```python
from build123d import *

# Parameters (mm, degrees)
SKETCH1_R           = 2.5
SKETCH1_R_2         = 1.75
SKETCH1_W           = 30
SKETCH1_H           = 6.4
BOSS_EXTRUDE1_DEPTH = 3.2


with BuildPart() as part:
    # Sketch1 → Boss-Extrude1 (new body)
    with BuildSketch(Plane(origin=(0, 0, 0), x_dir=(1, 0, 0), z_dir=(0, 1, 0))):
        Polygon((-87.5, 7.5), (-87.5, 20), (-84.3, 20), (-84.3, 35), (-87.5, 35), (-87.5, 50), (-70, 50), (-70, 46.8), (-50, 46.8), (-50, 50), (-30, 50), (-30, 46.8), (-10, 46.8), (-10, 50), (10, 50), (10, 46.8), (30, 46.8), (30, 50), (50, 50), (50, 46.8), (70, 46.8), (70, 50), (87.5, 50), (87.5, 35), (84.3, 35), (84.3, 20), (87.5, 20), (87.5, 7.5), (84.3, 7.5), (84.3, -7.5), (87.5, -7.5), (87.5, -20), (84.3, -20), (84.3, -35), (87.5, -35), (87.5, -50), (70, -50), (70, -46.8), (50, -46.8), (50, -50), (30, -50), (30, -46.8), (10, -46.8), (10, -50), (-10, -50), (-10, -46.8), (-30, -46.8), (-30, -50), (-50, -50), (-50, -46.8), (-70, -46.8), (-70, -50), (-87.5, -50), (-87.5, -35), (-84.3, -35), (-84.3, -20), (-87.5, -20), (-87.5, -7.5), (-84.3, -7.5), (-84.3, 7.5), align=None)
        with Locations((52.5, 15)):
            Circle(SKETCH1_R, mode=Mode.SUBTRACT)
        with Locations((42.34, 28)):
            Circle(SKETCH1_R_2, mode=Mode.SUBTRACT)
        with Locations((62.66, 28)):
            Circle(SKETCH1_R_2, mode=Mode.SUBTRACT)
        with Locations((62.66, -28)):
            Circle(SKETCH1_R_2, mode=Mode.SUBTRACT)
        with Locations((42.34, -28)):
            Circle(SKETCH1_R_2, mode=Mode.SUBTRACT)
        with Locations((52.5, -15)):
            Circle(SKETCH1_R, mode=Mode.SUBTRACT)
        with Locations((-54.3, 0)):
            Rectangle(SKETCH1_W, SKETCH1_H, mode=Mode.SUBTRACT)
    extrude(amount=BOSS_EXTRUDE1_DEPTH)


solid = part.part
```
Work out the finished part from the listing and answer in its coordinate system (mm). A direction names the side the tool comes from. Coordinates: 2 decimals unless noted, no trailing zeros. Loops run counter-clockwise (first coordinate to the right, second up) from the corner with the lowest first, then second, coordinate; pieces in that order, holes last. Notation, with made-up numbers: M 85.25,-38.75 L 143.25,-38.75 A27 ccw 143.25,-11.75 Z; hole C 31.5,5 d8. An arc over 180 degrees is marked long. Use CSV: the item, a comma, the result in double quotes. Start each with the question number.
(1) Find section A-A, the plane x = -63. Give the vertices of the cut face in (y, z), then the cut area to 3 significant figures.
(2) Find section B-B, the plane x = 62.66. Give the vertices of the cut face in (y, z), then the cut area to 3 significant figures.
(3) For faces 1 (the face through (10, 2, -48)), 2 (the face through (-69.3, 2, 0)), 3 (the face through (-84.3, 2, 0)), 4 (the face through (84.3, 2, -28)), determine the directions among +Z, -Z, +X, -X, +Y, -Y from which every point of the face is accessible in a straight line to the end or side of a thin tool.
(4) Given pin 1 Ø1.6 at (x, y) = (-51.5, 2) entering from -Z, flat-ended and moving along its own axis, determine where the tip first touches the part or whether it passes through.
(5) Consider line 1 (X direction, y = 1.8, z = -28); line 2 (Z direction, x = 62.66, y = 1.95); line 3 (Z direction, x = 52.5, y = 1.3). Determine where each line is inside the solid, lowest interval first.
(6) Find section C-C, the plane z = 15. Give the vertices of the cut face in (x, y).
(7) Find section D-D, the plane x = 42.34. Give the vertices of the cut face in (y, z), then the cut area to 3 significant figures.
(8) For a pull along Z with two mould halves and no side action, classify faces 5 (the face through (1, 0, -1)), 6 (the face through (0, 2, 50)), 7 (the face through (86, 2, -7.5)) as +Z half, -Z half, draft (parallel to the pull), parting line (faces both ways), or undercut.
Recorded:
1,outline,"M 0,-46.8 L 3.2,-46.8 L 3.2,-3.2 L 0,-3.2 Z; M 0,3.2 L 3.2,3.2 L 3.2,46.8 L 0,46.8 Z"
1,area,"279 mm^2"
2,outline,"M 0,-46.8 L 3.2,-46.8 L 3.2,-29.75 L 0,-29.75 Z; M 0,-26.25 L 3.2,-26.25 L 3.2,26.25 L 0,26.25 Z; M 0,29.75 L 3.2,29.75 L 3.2,46.8 L 0,46.8 Z"
2,area,"277 mm^2"
3,face 1,"-Z, +Y, -Y"
3,face 2,"+Y, -Y"
3,face 3,"-X, +Y, -Y"
3,face 4,"+X, +Y, -Y"
4,pin 1,"stops at z = -46.8"
5,line 1,"x = -84.3 to 40.59, 44.09 to 60.91, 64.41 to 84.3"
5,line 2,"z = -46.8 to -29.75, -26.25 to 26.25, 29.75 to 46.8"
5,line 3,"z = -46.8 to -17.5, -12.5 to 12.5, 17.5 to 46.8"
6,outline,"M -87.5,0 L 50,0 L 50,3.2 L -87.5,3.2 Z; M 55,0 L 87.5,0 L 87.5,3.2 L 55,3.2 Z"
7,outline,"M 0,-50 L 3.2,-50 L 3.2,-29.75 L 0,-29.75 Z; M 0,-26.25 L 3.2,-26.25 L 3.2,26.25 L 0,26.25 Z; M 0,29.75 L 3.2,29.75 L 3.2,50 L 0,50 Z"
7,area,"298 mm^2"
8,face 5,"draft"
8,face 6,"+Z half"
8,face 7,"undercut"
